from build123d import *

# Parameters (mm, degrees)
SKETCH_1_W                       = 150
SKETCH_1_H                       = 150
EXTRUDE_1_DEPTH                  = 5.5
SKETCH_2_R                       = 2.5
CUT_EXTRUDE_1_DEPTH              = 107.208521315
CUT_EXTRUDE_2_DEPTH              = 107.208521315
CUT_EXTRUDE_2_DEPTH_BACK         = 107.208521315
SKETCH_3_R                       = 55
PATTERN_CIRCULAR_1_COUNT         = 4
SKETCH_4_R                       = 1.6
CUT_EXTRUDE_3_DEPTH              = 107.208521315
CHAMFER_1_SIZE                   = 40
CHAMFER_2_SIZE                   = 40
PATTERN_LINEAR_1_COUNT           = 2
PATTERN_LINEAR_1_PITCH           = 90
PATTERN_LINEAR_2_COPY_1_SKETCH_R = 1.6
PATTERN_LINEAR_2_COPY_1_DEPTH    = 107.208521315
PATTERN_LINEAR_2_COPY_2_SKETCH_R = 1.6
PATTERN_LINEAR_2_COPY_2_DEPTH    = 107.208521315


with BuildPart() as part:
    # ｽｹｯﾁ1 → ﾎﾞｽ - 押し出し1 (new body)
    with BuildSketch(Plane.XY):
        Rectangle(SKETCH_1_W, SKETCH_1_H)
    extrude(amount=EXTRUDE_1_DEPTH)

    # ｽｹｯﾁ2 → ｶｯﾄ - 押し出し1 (cut, symmetric)
    with BuildSketch(Plane(origin=(0, 0, 0), x_dir=(-1, 0, 0), z_dir=(0, 0, -1))):
        with Locations((-45.254833996, -45.254833996)):
            Circle(SKETCH_2_R)
    cut_extrude_1 = extrude(amount=CUT_EXTRUDE_1_DEPTH, both=True, mode=Mode.SUBTRACT)

    # ｽｹｯﾁ3 → ｶｯﾄ - 押し出し2 (cut, two sides: drawn at the far end of the back side and taken through both)
    with BuildSketch(Plane(origin=(0, 0, 0), x_dir=(-1, 0, 0), z_dir=(0, 0, -1)).offset(-CUT_EXTRUDE_2_DEPTH_BACK)):
        Circle(SKETCH_3_R)
    extrude(amount=CUT_EXTRUDE_2_DEPTH + CUT_EXTRUDE_2_DEPTH_BACK, mode=Mode.SUBTRACT)

    # 円形ﾊﾟﾀｰﾝ1: ｶｯﾄ - 押し出し1 ×4 about axis
    pattern_circular_1_axis = Axis((0, 0, 0), (0, 0, 1))
    for i in range(1, PATTERN_CIRCULAR_1_COUNT):
        add(cut_extrude_1.rotate(pattern_circular_1_axis, i * 360 / PATTERN_CIRCULAR_1_COUNT), mode=Mode.SUBTRACT)

    # ｽｹｯﾁ4 → ｶｯﾄ - 押し出し3 (cut, symmetric)
    with BuildSketch(Plane(origin=(0, 0, 0), x_dir=(-1, 0, 0), z_dir=(0, 0, -1))):
        with Locations((65, -65)):
            Circle(SKETCH_4_R)
    cut_extrude_3 = extrude(amount=CUT_EXTRUDE_3_DEPTH, both=True, mode=Mode.SUBTRACT)

    # 面取り1
    chamfer_1_edges = [part.edges().sort_by_distance(p)[0] for p in [
        (-75, 75, 2.75),
    ]]
    chamfer(chamfer_1_edges, length=CHAMFER_1_SIZE)

    # 面取り2
    chamfer_2_edges = [part.edges().sort_by_distance(p)[0] for p in [
        (75, -75, 2.75),
    ]]
    chamfer(chamfer_2_edges, length=CHAMFER_2_SIZE)

    # 直線ﾊﾟﾀｰﾝ1: ｶｯﾄ - 押し出し3 ×2
    with Locations(*[(0, i * PATTERN_LINEAR_1_PITCH, 0) for i in range(1, PATTERN_LINEAR_1_COUNT)]):
        add(cut_extrude_3, mode=Mode.SUBTRACT)

    # ﾐﾗｰ1: ｶｯﾄ - 押し出し3 across plane
    add(cut_extrude_3.mirror(Plane(origin=(0, 0, 0), x_dir=(0, 0, 1), z_dir=(-0.7071067811865475, -0.7071067811865476, 0))), mode=Mode.SUBTRACT)

    # 直線ﾊﾟﾀｰﾝ2 copy 1 sketch → 直線ﾊﾟﾀｰﾝ2 copy 1 (cut, symmetric)
    with BuildSketch(Plane(origin=(-90, 0, 0), x_dir=(0, 1, 0), z_dir=(0, 0, -1))):
        with Locations((65, 65)):
            Circle(PATTERN_LINEAR_2_COPY_1_SKETCH_R)
    extrude(amount=PATTERN_LINEAR_2_COPY_1_DEPTH, both=True, mode=Mode.SUBTRACT)

    # 直線ﾊﾟﾀｰﾝ2 copy 2 sketch → 直線ﾊﾟﾀｰﾝ2 copy 2 (cut, symmetric)
    with BuildSketch(Plane(origin=(-90, 0, 0), x_dir=(-1, 0, 0), z_dir=(0, 0, -1))):
        with Locations((65, -65)):
            Circle(PATTERN_LINEAR_2_COPY_2_SKETCH_R)
    extrude(amount=PATTERN_LINEAR_2_COPY_2_DEPTH, both=True, mode=Mode.SUBTRACT)


solid = part.part
The model under review builds one solid part; all positions refer to its coordinate system, in mm. Coordinates: 2 decimals unless noted, no trailing zeros. Loops run counter-clockwise (first coordinate to the right, second up) from the corner with the lowest first, then second, coordinate; pieces in that order, holes last.
(1) Draft analysis for pull direction Y (two halves, no side actions). For faces 1 (the flat face through (-21, -75, 3)), 2 (the cylindrical face through (-43.911, 43.147, 2.712)), 3 (the cylindrical face through (11.923, -53.692, 2.788)), 4 (the flat face through (32, 51, 0)), state which applies: +Y half, -Y half, draft (parallel to the pull), parting line (faces both ways), or undercut.
Determined:
face 1: -Y half
face 2: undercut
face 3: undercut
face 4: draft
(2) Consider section A-A, the plane x = 0. Give the boundary of the cut face in (y, z), plus the area to 3 significant figures.
Determined:
outline: (-75, 0) - (-55, 0) - (-55, 5.5) - (-75, 5.5) - close; (55, 0) - (75, 0) - (75, 5.5) - (55, 5.5) - close
area: 220 mm2
(3) Consider section D-D, the plane x = -57. Give the boundary of the cut face in (y, z), plus the area to 3 significant figures.
Determined:
outline: (-75, 0) - (53, 0) - (53, 5.5) - (-75, 5.5) - close
area: 704 mm2
(4) Consider section C-C, the plane z = 4.55. Give the number of separate pieces and of enclosed holes in the cut face, plus the area to 3 significant figures.
Determined:
separate pieces: 1
enclosed holes: 9
area: 11,300 mm2
(5) Wall thickness on L1, parallel to Y at x = 0, z = 1.3; L2, parallel to Y at x = -44, z = 4.8; L3, parallel to X at y = 1.5, z = 1.8: over which ranges is each line inside the solid? List them lowest first.
Determined:
L1: y = -75 to -55, 55 to 75
L2: y = -75 to -47.42, -43.09 to -33, 33 to 43.09, 47.42 to 66
L3: x = -75 to -54.98, 54.98 to 75
